Build history of the part. All positions in model axes, mm. A direction names the side the tool comes from. Round coordinates to 2 decimals unless told otherwise and drop trailing zeros. Write each loop counter-clockwise with the first axis right and the second up, starting at its lowest first coordinate (ties: lowest second). Pieces come first, ordered by that corner, then holes. Notation, with made-up numbers: (71.5, 39.25) - (81.5, 39.25) arc R31 ccw to (81.5, 72.25) - close; hole circle Ø6 at (-31, -2). An arc over 180 degrees is marked (long way). Answer as a JSON object with one key per item and string values. Group by question number.
Item 1: Probe line 1 (Y direction, x = 6, z = 3.9); line 2 (Y direction, x = 2.75, z = 4.05); line 3 (Z direction, x = 1, y = -59). List the from-to ranges inside material, lowest first. Write a range as from..to.
Item 2: Slice it at B-B, the plane y = -64. List the corners of the cut face in (x, z), then the cut area to 3 significant figures.
Item 3: Flat gauge pins, fed straight in: pin 1 (0.5 mm diameter, centred on x = 3.5, z = 1.5, fed in from -Y); pin 2 (2.5 mm diameter, centred on x = 3.5, y = -1.5, fed in from +Z); pin 3 (0.6 mm diameter, centred on x = 2.5, z = 3, fed in from +Y). Where does each tip first touch, or does it go through?
Item 4: Which spindle directions (+Z, -Z, +X, -X, +Y, -Y) get a long thin tool onto all of the face, cutting with end or side? Do faces 4 (the flat face through (3, -1, 2)), 5 (the flat face through (0, -82, 1)). Say none if no direction does.
Item 5: Slice it at A-A, the plane x = 4.5. List the corners of the cut face in (y, z), then the cut area to 3 significant figures.
Item 6: Two-plate mould, pull along Y, no slides. Class faces 1 (the cylindrical face through (3.2, -159, 2.4)), 2 (the flat face through (3, -79, 2)), 3 (the cylindrical face through (3.16, -161.14, 0.9)): +Y half, -Y half, draft (parallel to the pull), parting line (faces both ways), or undercut.
from build123d import *

# Parameters (mm, degrees)
F1_DEPTH = 6.4


# Not quite as in the source:
# - a feature names something its author has since deleted; it is built from what else it names


with BuildPart() as f1:
    # F0 (on Right) → F1 (new body)
    with BuildSketch(Plane.YZ):
        with BuildLine():
            Line((-159, 0), (0, 0))
            Line((0, 0), (0, 2))
            Line((0, 2), (-3, 2))
            Line((-3, 2), (-3, 1))
            Line((-3, 1), (-5, 1))
            Line((-5, 1), (-5, 2))
            Line((-5, 2), (-156, 2))
            Line((-156, 2), (-156, 3.9))
            ThreePointArc((-156, 3.9), (-156.1464466094, 4.2535533906), (-156.5, 4.4))
            Line((-156.5, 4.4), (-156.5505102572, 4.4))
            ThreePointArc((-156.5505102572, 4.4), (-156.8667380232, 4.2872983346), (-157.0404082058, 4))
            ThreePointArc((-157.0404082058, 4), (-159, 2.4), (-160.9595917942, 4))
            ThreePointArc((-160.9595917942, 4), (-161.1332619768, 4.2872983346), (-161.4494897428, 4.4))
            Line((-161.4494897428, 4.4), (-161.5, 4.4))
            ThreePointArc((-161.5, 4.4), (-161.8535533906, 4.2535533906), (-162, 3.9))
            Line((-162, 3.9), (-162, 3))
            ThreePointArc((-162, 3), (-161.1213203436, 0.8786796564), (-159, 0))
        make_face()
    extrude(amount=F1_DEPTH)


solid = f1.part
Geometry says:
{
 "1": {"line 1": "y = -162..-160.94, -157.06..-156", "line 2": "y = -161.98..-160.97, -157.03..-156.02", "line 3": "z = 0..2"},
 "2": {"outline": "(0, 0) - (6.4, 0) - (6.4, 2) - (0, 2) - close", "area": "12.8 mm^2"},
 "3": {"pin 1": "stops at y = -161.73", "pin 2": "stops at z = 2", "pin 3": "stops at y = -156"},
 "4": {"face 4": "+Z, +X, -X, +Y", "face 5": "+Z, -Z, -X, +Y, -Y"},
 "5": {"outline": "(-162, 3) arc R3 ccw to (-159, 0) - (0, 0) - (0, 2) - (-3, 2) - (-3, 1) - (-5, 1) - (-5, 2) - (-156, 2) - (-156, 3.9) arc R0.5 ccw to (-156.5, 4.4) - (-156.55, 4.4) arc R0.5 ccw to (-157.04, 4) arc R2 cw to (-160.96, 4) arc R0.5 ccw to (-161.45, 4.4) - (-161.5, 4.4) arc R0.5 ccw to (-162, 3.9) - close", "area": "328 mm^2"},
 "6": {"face 1": "undercut", "face 2": "draft", "face 3": "-Y half"}
}
